Geometry: final body of the model. Coordinates: model frame, mm. Face numbers are marked on the shaded views. A direction names the side the tool comes from. Round coordinates to 2 decimals unless told otherwise and drop trailing zeros. Loops run counter-clockwise (first coordinate to the right, second up) from the corner with the lowest first, then second, coordinate; pieces in that order, holes last. Notation, with made-up numbers: (86.25, 36) - (110.25, 36) arc R19 ccw to (110.25, 55) - close; hole circle Ø5 at (51.5, 39.25). An arc over 180 degrees is marked (long way). Return JSON: item names as keys, results as strings. Group by question number.
1. Section D-D on x = -16. Return loops of the section in (y, z).
2. Section B-B on x = 14. Return loops of the section in (y, z), and give its area (3 significant figures).
3. Material intervals for probe 1 along X at (y, z) = (-3.5, 4); probe 2 along Y at (x, z) = (19, 7); probe 3 along Y at (x, z) = (0, 2.75), sorted ascending.
4. Draft query along X for the marked faces 3, 4, 5 and 6. Return one class per face: +X half, -X half, draft (parallel to the pull), parting line (faces both ways), or undercut.
5. Set-up query: the marked faces 1 and 2. Return all of +Z, -Z, +X, -X, +Y, -Y with unobstructed straight access to the full face (end or side cutting, diameter ignored); none if empty.
6. First-contact query: pin 1 Ø4 at (x, y) = (14.5, 0) entering from +Z; pin 2 Ø3 at (y, z) = (-2.5, 5.5) entering from +X; pin 3 Ø1 at (y, z) = (-1, 5) entering from -X. Flat tips, straight axial feed; report the tip coordinate or a pass-through.
7. Section C-C on y = -1. Return loops of the section in (x, z), and give its area (3 significant figures).
8. Section A-A on z = 4. Count the separate pieces of the cut face and the enclosed holes in it, and give its area (3 significant figures).
from build123d import *

# Parameters (mm, degrees)
BOSS_EXTRUDE1_DEPTH        = 10
M3X0_5_TAPPED_HOLE1_D      = 2.5
M3X0_5_TAPPED_HOLE1_DEPTH  = 3.74999984
M3X0_5_TAPPED_HOLE2_D      = 3
F_3_0MM_DOWEL_HOLE1_REACH  = 40.325
F_3_0MM_DOWEL_HOLE1_BORE_R = 1.5


with BuildPart() as part:
    # Sketch1 → Boss-Extrude1 (new body)
    with BuildSketch(Plane.XY):
        with BuildLine():
            Line((-19.997736867, 0.25), (-11.98520546, 0.25))
            ThreePointArc((-11.98520546, 0.25), (-6.997736867, 0), (-11.98520546, -0.25))
            Line((-11.98520546, -0.25), (-20, -0.25))
            Line((-20, -0.25), (-19.997736867, -3.99999984))
            Line((-19.997736867, -3.99999984), (19.997736867, -3.99999984))
            Line((19.997736867, -3.99999984), (19.997736867, -0.25))
            Line((19.997736867, -0.25), (11.98520546, -0.25))
            ThreePointArc((11.98520546, -0.25), (6.997736867, 0), (11.98520546, 0.25))
            Line((11.98520546, 0.25), (19.997736867, 0.25))
            Line((19.997736867, 0.25), (20.997736867, 0.25))
            Line((20.997736867, 0.25), (20.997736867, 3.99999984))
            Line((20.997736867, 3.99999984), (20.002263133, 3.99999984))
            Line((20.002263133, 3.99999984), (-19.997736867, 3.99999984))
            Line((-19.997736867, 3.99999984), (-20.997736867, 3.99999984))
            Line((-20.997736867, 3.99999984), (-20.997736867, 0.25))
            Line((-20.997736867, 0.25), (-19.997736867, 0.25))
        make_face()
    extrude(amount=BOSS_EXTRUDE1_DEPTH)

    # M3x0.5 Tapped Hole1
    with Locations(Plane(origin=(-16, -3.99999984, 4), x_dir=(-1, 0, 0), z_dir=(0, -1, 0))):
        with Locations((0, 0), (-32, 0)):
            Hole(M3X0_5_TAPPED_HOLE1_D / 2, depth=M3X0_5_TAPPED_HOLE1_DEPTH)

    # M3x0.5 Tapped Hole2 (through all)
    with Locations(Plane.XY.offset(10)):
        with Locations((0, 0)):
            Hole(M3X0_5_TAPPED_HOLE2_D / 2)

    # Ø3.0mm Dowel Hole1 bore (on position points) → Ø3.0mm Dowel Hole1 (cut, up to next)
    with BuildSketch(Plane(origin=(16, 3.99999984, 4), x_dir=(0, 0, 1), z_dir=(0, 1, 0)), mode=Mode.PRIVATE) as f_3_0mm_dowel_hole1_sk1:
        Circle(F_3_0MM_DOWEL_HOLE1_BORE_R)
    f_3_0mm_dowel_hole1_tool1 = extrude(f_3_0mm_dowel_hole1_sk1.sketch, amount=-F_3_0MM_DOWEL_HOLE1_REACH, mode=Mode.PRIVATE) & part.part
    # Ø3.0mm Dowel Hole1 bore (on position points) → Ø3.0mm Dowel Hole1 (cut, up to next)
    with BuildSketch(Plane(origin=(16, 3.99999984, 4), x_dir=(0, 0, 1), z_dir=(0, 1, 0)), mode=Mode.PRIVATE) as f_3_0mm_dowel_hole1_sk2:
        with Locations((0, -32)):
            Circle(F_3_0MM_DOWEL_HOLE1_BORE_R)
    f_3_0mm_dowel_hole1_tool2 = extrude(f_3_0mm_dowel_hole1_sk2.sketch, amount=-F_3_0MM_DOWEL_HOLE1_REACH, mode=Mode.PRIVATE) & part.part
    add(f_3_0mm_dowel_hole1_tool1.solids().sort_by_distance((16, 4, 4))[0], mode=Mode.SUBTRACT)
    add(f_3_0mm_dowel_hole1_tool2.solids().sort_by_distance((-16, 4, 4))[0], mode=Mode.SUBTRACT)


solid = part.part
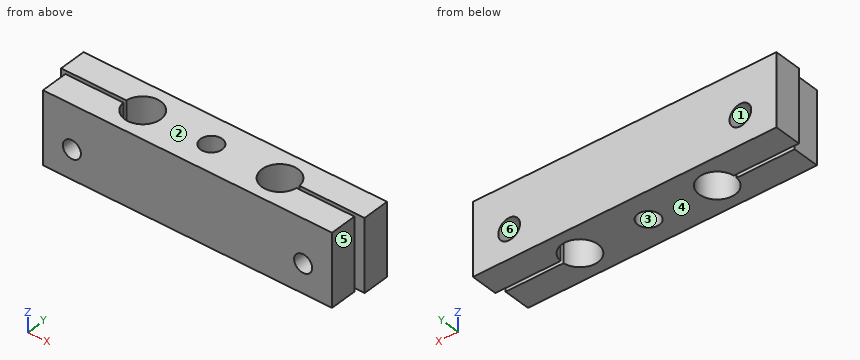
Taken from the geometry:
{
 "1": {"outline": "(-4, 0) - (-0.25, 0) - (-0.25, 2.75) - (-4, 2.75) - close; (-4, 5.25) - (-0.25, 5.25) - (-0.25, 10) - (-4, 10) - close; (0.25, 0) - (4, 0) - (4, 2.5) - (0.25, 2.5) - close; (0.25, 5.5) - (4, 5.5) - (4, 10) - (0.25, 10) - close"},
 "2": {"outline": "(-4, 0) - (-0.25, 0) - (-0.25, 10) - (-4, 10) - close; (0.25, 0) - (4, 0) - (4, 10) - (0.25, 10) - close", "area": "75.0 mm2"},
 "3": {"probe 1": "-20 to -17.25, -14.75 to 14.75, 17.25 to 20", "probe 2": "-4 to -0.25, 0.25 to 4", "probe 3": "-4 to -1.5, 1.5 to 4"},
 "4": {"face 3": "undercut", "face 4": "draft", "face 5": "+X half", "face 6": "undercut"},
 "5": {"face 1": "+Y", "face 2": "+Z, +X, -X, +Y, -Y"},
 "6": {"pin 1": "z = 10", "pin 2": "x = 20", "pin 3": "x = -20"},
 "7": {"outline": "(-20, 0) - (-11.79, 0) - (-11.79, 10) - (-20, 10) - close; (-7.21, 0) - (-1.12, 0) - (-1.12, 10) - (-7.21, 10) - close; (1.12, 0) - (7.21, 0) - (7.21, 10) - (1.12, 10) - close; (11.79, 0) - (20, 0) - (20, 10) - (11.79, 10) - close; hole circle Ø2.5 at (-16, 4); hole circle Ø2.5 at (16, 4)", "area": "276 mm2"},
 "8": {"separate pieces": "5", "enclosed holes": "1", "area": "232 mm2"}
}
